from build123d import *

# Parameters (mm, degrees)
SKETCH1_W              = 150
SKETCH1_H              = 30
SKETCH1_W_2            = 80
SKETCH1_H_2            = 15
BOSS_EXTRUDE1_DEPTH    = 145
CUT_EXTRUDE1_DEPTH     = 145
CUT_EXTRUDE2_DEPTH     = 15
CUT_EXTRUDE3_DEPTH     = 10
M20_TAPPED_HOLE1_D     = 17.5
M20_TAPPED_HOLE1_DEPTH = 40
M20_TAPPED_HOLE1_TIP   = 5.257530416
SKETCH7_R              = 5
CUT_EXTRUDE4_DEPTH     = 83
SKETCH8_R              = 55
CUT_EXTRUDE5_DEPTH     = 15


with BuildPart() as part:
    # Sketch1 → Boss-Extrude1 (new body)
    with BuildSketch(Plane.XY):
        with Locations((75, 15)):
            Rectangle(SKETCH1_W, SKETCH1_H)
        with Locations((75, 37.5)):
            Rectangle(SKETCH1_W_2, SKETCH1_H_2)
    extrude(amount=BOSS_EXTRUDE1_DEPTH)

    # Sketch2 → Cut-Extrude1 (cut)
    with BuildSketch(Plane(origin=(0, 0, 0), x_dir=(1, 0, 0), z_dir=(0, 1, 0))):
        with BuildLine():
            Line((72.5, 0), (0, 0))
            Line((0, 0), (0, -72.5))
            ThreePointArc((0, -72.5), (21.234758364, -21.234758364), (72.5, 0))
        make_face()
        with BuildLine():
            ThreePointArc((72.5, -145), (21.234758364, -123.765241636), (0, -72.5))
            Line((0, -72.5), (0, -145))
            Line((0, -145), (72.5, -145))
        make_face()
        with BuildLine():
            Line((150, 0), (72.5, 0))
            ThreePointArc((72.5, 0), (123.765241636, -21.234758364), (145, -72.5))
            ThreePointArc((145, -72.5), (123.765241636, -123.765241636), (72.5, -145))
            Line((72.5, -145), (150, -145))
            Line((150, -145), (150, 0))
        make_face()
    extrude(amount=CUT_EXTRUDE1_DEPTH, mode=Mode.SUBTRACT)

    # Sketch3 → Cut-Extrude2 (cut)
    with BuildSketch(Plane(origin=(0, 45, 0), x_dir=(1, 0, 0), z_dir=(0, 1, 0))):
        with BuildLine():
            ThreePointArc((115, -13.763299378), (75.498630618, -0.062038858), (35, -10.45163177))
            Line((35, -10.45163177), (35, -72.50163177))
            ThreePointArc((35, -72.50163177), (75, -32.50163177), (115, -72.50163177))
            Line((115, -72.50163177), (115, -13.763299378))
        make_face()
        with BuildLine():
            ThreePointArc((115, -72.50163177), (75, -112.50163177), (35, -72.50163177))
            Line((35, -72.50163177), (35, -134.54836823))
            ThreePointArc((35, -134.54836823), (75.498630618, -144.937961142), (115, -131.236700622))
            Line((115, -131.236700622), (115, -72.50163177))
        make_face()
    extrude(amount=-CUT_EXTRUDE2_DEPTH, mode=Mode.SUBTRACT)

    # Sketch4 → Cut-Extrude3 (cut)
    with BuildSketch(Plane(origin=(0, 45, 0), x_dir=(1, 0, 0), z_dir=(0, 1, 0))):
        with BuildLine():
            Line((55, -107.142647921), (55, -72.142647921))
            ThreePointArc((55, -72.142647921), (75, -52.498410294), (95, -72.142647921))
            Line((95, -72.142647921), (95, -107.142647921))
            ThreePointArc((95, -107.142647921), (75, -112.50163177), (55, -107.142647921))
        make_face()
    extrude(amount=-CUT_EXTRUDE3_DEPTH, mode=Mode.SUBTRACT)

    # M20 Tapped Hole1
    with Locations(Plane(origin=(75, 35, 72.50163177), x_dir=(0, 0, 1), z_dir=(0, 1, 0))):
        with Locations((0, 0)):
            Hole(M20_TAPPED_HOLE1_D / 2, depth=M20_TAPPED_HOLE1_DEPTH)
            with Locations((0, 0, -(M20_TAPPED_HOLE1_DEPTH + M20_TAPPED_HOLE1_TIP / 2))):  # 118° drill point
                Cone(0, M20_TAPPED_HOLE1_D / 2, M20_TAPPED_HOLE1_TIP, mode=Mode.SUBTRACT)

    # Sketch7 → Cut-Extrude4 (cut)
    with BuildSketch(Plane(origin=(0, 0, 0), x_dir=(1, 0, 0), z_dir=(0, 1, 0))):
        with Locations((74.583225581, -127.50163177)):
            Circle(SKETCH7_R)
        with Locations((27.368602792, -45.00163177)):
            Circle(SKETCH7_R)
        with Locations((122.631397208, -45.00163177)):
            Circle(SKETCH7_R)
    extrude(amount=CUT_EXTRUDE4_DEPTH, mode=Mode.SUBTRACT)

    # Sketch8 → Cut-Extrude5 (cut)
    with BuildSketch(Plane.XZ):
        with Locations((75, 72.50163177)):
            Circle(SKETCH8_R)
    extrude(amount=-CUT_EXTRUDE5_DEPTH, mode=Mode.SUBTRACT)


solid = part.part
Here's how the part is built. I have some questions about the finished solid (model axes, mm). A direction names the side the tool comes from. Coordinates: 2 decimals unless noted, no trailing zeros. Order: outer loops, then holes, each group sorted by start corner. A loop starts at its lowest first (then second) coordinate and runs counter-clockwise, first axis right, second up. Notation, with made-up numbers: (-1, 54) -> (47, 54) arc R10 ccw to (47, 73) -> close; hole circle Ø2 at (-14, 44.5). An arc over 180 degrees is marked (long way). Answer in a Markdown table with one row per item.
(1) I want a section at A-A on x = 75. List the corners of the cut face in (y, z) for me.
Answer key:
| item | result |
|---|---|
| outline | (0, 0.04) -> (30, 0.04) -> (30, 32.5) -> (45, 32.5) -> (45, 52.5) -> (35, 52.5) -> (35, 63.75) -> (15, 63.75) -> (15, 17.5) -> (0, 17.5) -> close; (0, 132.48) -> (30, 132.48) -> (30, 144.96) -> (0, 144.96) -> close; (15, 81.25) -> (35, 81.25) -> (35, 112.5) -> (30, 112.5) -> (30, 122.52) -> (15, 122.52) -> close |
(2) Will these pins go through, and if not, where does the flat tip stop? pin 1 Ø4 at (y, z) = (22, 107) entering from +X; pin 2 Ø11 at (y, z) = (38.5, 95.5) entering from -X; pin 3 Ø3 at (y, z) = (27, 90) entering from +X.
Answer key:
| item | result |
|---|---|
| pin 1 | x = 137.31 |
| pin 2 | x = 39.03 |
| pin 3 | x = 143.21 |
(3) On a 3-axis mill with a long thin cutter (end or side, diameter ignored), from which of +Z, -Z, +X, -X, +Y, -Y can I reach the whole of each face in a straight line? I mean faces 1 (the face through (27.633, 7.395, 100.455)), 2 (the face through (74.565, 40.07, 52.503)), 3 (the face through (73.499, 18.123, 132.383)). Say none if no direction works.
Answer key:
| item | result |
|---|---|
| face 1 | -Y |
| face 2 | +Z, +Y |
| face 3 | +Y, -Y |
(4) Thinking about a two-plate mould opening in Z: for faces 4 (the face through (104, 30, 104)), 5 (the face through (83.676, 24.86, 73.641)), 6 (the face through (74.264, 7.395, 17.507)), 7 (the face through (80.207, 37.605, 32.842)), which applies, +Z half, -Z half, draft (parallel to the pull), parting line (faces both ways), or undercut?
Answer key:
| item | result |
|---|---|
| face 4 | draft |
| face 5 | undercut |
| face 6 | undercut |
| face 7 | parting line |
(5) I want a section at D-D on x = 122.5. List the corners of the cut face in (y, z) for me, then the cut area to 3 significant figures.
Answer key:
| item | result |
|---|---|
| outline | (0, 20) -> (30, 20) -> (30, 40) -> (0, 40) -> close; (0, 100.23) -> (15, 100.23) -> (15, 50) -> (30, 50) -> (30, 125) -> (0, 125) -> close |
| area | 2,100 mm^2 |
(6) I want a section at C-C on y = 13. List the corners of the cut face in (x, z) for me, then the cut area to 3 significant figures.
Answer key:
| item | result |
|---|---|
| outline | circle Ø145 at (72.5, 72.5); hole (25.07, 49.44) arc R5 ccw (long way) to (30.06, 40.79) arc R55 ccw to (119.94, 40.79) arc R5 ccw (long way) to (124.93, 49.44) arc R55 ccw to (79.58, 127.31) arc R5 ccw (long way) to (69.59, 127.23) arc R55 ccw to start |
| area | 6,890 mm^2 |
(7) Please list where these lines run through material, in increasing order: probe 1 along Y at (x, z) = (46.5, 92); probe 2 along X at (y, z) = (41, 78); probe 3 along X at (y, z) = (3, 113.5).
Answer key:
| item | result |
|---|---|
| probe 1 | 15 to 45 |
| probe 2 | 35.38 to 55, 95 to 114.62 |
| probe 3 | 12.71 to 38.34, 111.66 to 132.29 |
(8) I want a section at B-B on z = 65.5. List the corners of the cut face in (x, y) for me, then the cut area to 3 significant figures.
Answer key:
| item | result |
|---|---|
| outline | (0.34, 0) -> (20.45, 0) -> (20.45, 15) -> (69.75, 15) -> (69.75, 35) -> (56.26, 35) -> (56.26, 45) -> (35.62, 45) -> (35.62, 30) -> (0.34, 30) -> close; (80.25, 15) -> (129.55, 15) -> (129.55, 0) -> (144.66, 0) -> (144.66, 30) -> (114.38, 30) -> (114.38, 45) -> (93.74, 45) -> (93.74, 35) -> (80.25, 35) -> close |
| area | 3,290 mm^2 |
